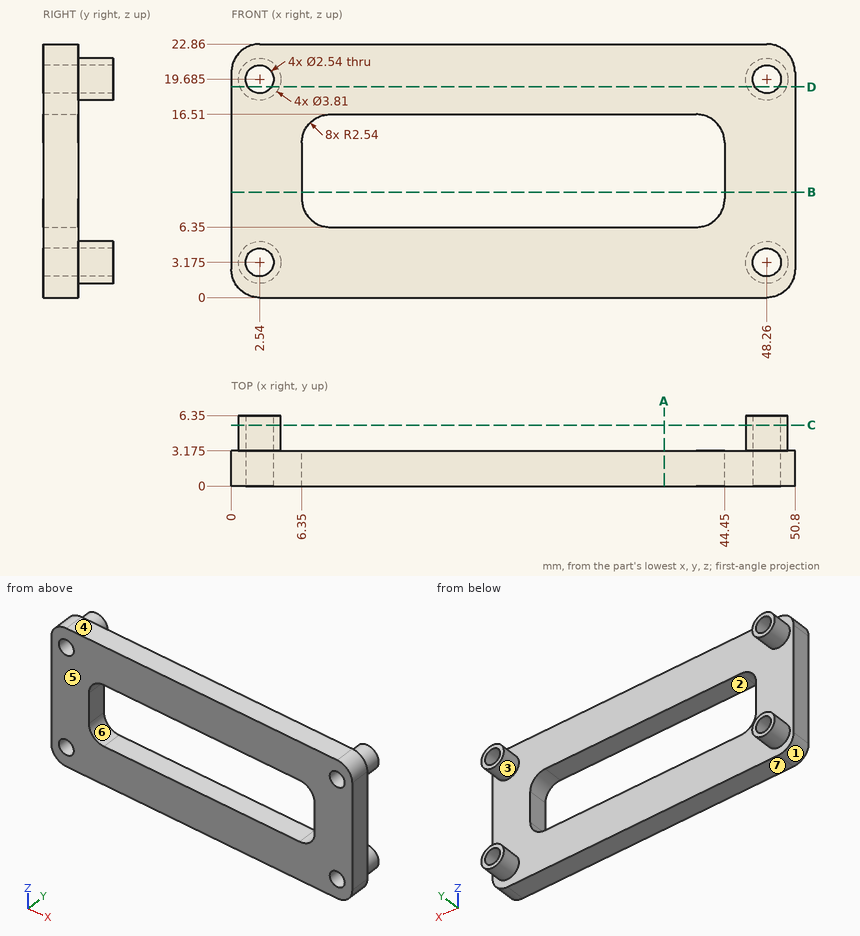
Geometry check sheet. Reference: drawing and pictorial views, mm from the part's lowest x, y, z. A direction names the side the tool comes from. Round coordinates to 2 decimals unless told otherwise and drop trailing zeros. Order: outer loops, then holes, each group sorted by start corner. A loop starts at its lowest first (then second) coordinate and runs counter-clockwise, first axis right, second up. Notation, with made-up numbers: (-39.5, 19.5) - (-8.5, 19.5) arc R14 cw to (-8.5, 32.5) - close; hole circle Ø11 at (53.25, -21.75). An arc over 180 degrees is marked (long way). Use a Markdown table: item, result. Add a question column.
1) Section check C-C (y = 5.5). Record the cut outline in (x, z) (3 decimals).
2) Thickness scan on line 1 along Z through (x, y) = (2.54, 2.25) (3 decimals); line 2 along Z through (x, y) = (48.26, 4) (3 decimals); line 3 along X through (y, z) = (1, 2.25). Record the ranges inside material, lowest first.
3) Set-up check for the marked faces 1, 2 and 3: record each of +Z, -Z, +X, -X, +Y, -Y from which the full face is reachable in a straight line by a thin tool's end or side.
4) Mould release check, pull along Z, two halves, no side actions. Record for the marked faces 4, 5, 6 and 7: released by +Z, released by -Z, zero draft, split by the parting line, or undercut.
5) Gauge pin test, flat ends, axial feed: P1, Ø5, axis at x = 13, z = 18.5, coming from the +Y side (3 decimals); P2, Ø2, axis at x = 32.5, z = 14, coming from the -Y side; P3, Ø1, axis at y = 4, z = 18.5, coming from the -X side. Record the tip position at first contact, or that the pin passes through.
6) Section check B-B (z = 9.5). Record the cut outline in (x, y) (3 decimals), then the cut area to 3 significant figures.
7) Section check A-A (x = 39). Record the cut outline in (y, z) (3 decimals).
8) Section check D-D (z = 19). Record the cut outline in (x, y) (3 decimals).
Established:
| question | item | result |
|---|---|---|
| 1 | outline | circle Ø3.81 at (2.54, 3.175); circle Ø3.81 at (2.54, 19.685); circle Ø3.81 at (48.26, 3.175); circle Ø3.81 at (48.26, 19.685); hole circle Ø2.54 at (2.54, 3.175); hole circle Ø2.54 at (2.54, 19.685); hole circle Ø2.54 at (48.26, 3.175); hole circle Ø2.54 at (48.26, 19.685) |
| 2 | line 1 | 0 to 1.905, 4.445 to 18.415, 20.955 to 22.86 |
| 2 | line 2 | 1.27 to 1.905, 4.445 to 5.08, 17.78 to 18.415, 20.955 to 21.59 |
| 2 | line 3 | 0.02 to 1.67, 3.41 to 47.39, 49.13 to 50.78 |
| 3 | face 1 | -Z, -X, +Y, -Y |
| 3 | face 2 | +Y, -Y |
| 3 | face 3 | +Y |
| 4 | face 4 | released by +Z |
| 4 | face 5 | zero draft |
| 4 | face 6 | undercut |
| 4 | face 7 | released by -Z |
| 5 | P1 | y = 3.175 |
| 5 | P2 | through |
| 5 | P3 | x = 0.76 |
| 6 | outline | (0, 0) - (6.35, 0) - (6.35, 3.175) - (0, 3.175) - close; (44.45, 0) - (50.8, 0) - (50.8, 3.175) - (44.45, 3.175) - close |
| 6 | area | 40.3 mm2 |
| 7 | outline | (0, 0) - (3.175, 0) - (3.175, 6.35) - (0, 6.35) - close; (0, 16.51) - (3.175, 16.51) - (3.175, 22.86) - (0, 22.86) - close |
| 8 | outline | (0, 0) - (1.471, 0) - (1.471, 6.35) - (0.762, 6.35) - (0.762, 3.175) - (0, 3.175) - close; (3.609, 0) - (47.191, 0) - (47.191, 6.35) - (46.482, 6.35) - (46.482, 3.175) - (4.318, 3.175) - (4.318, 6.35) - (3.609, 6.35) - close; (49.329, 0) - (50.8, 0) - (50.8, 3.175) - (50.038, 3.175) - (50.038, 6.35) - (49.329, 6.35) - close |
